Autodesk Inventor part; units mm, degrees
ref_plane "YZ Plane" through (0, 0, 0) normal (1, 0, 0) x (0, 1, 0)
ref_plane "XZ Plane" through (0, 0, 0) normal (0, 1, 0) x (-1, 0, 0)
ref_plane "XY Plane" through (0, 0, 0) normal (0, 0, 1) x (1, 0, 0)
sketch "Boceto1" plane through (0, 0, 0) normal (0, 1, 0) x (-1, 0, 0)
  circle A0 centre (0, 0) radius 15
  dimension "d0" = 30
extrude "Extrusión1" add sketch "Boceto1" along normal blind 4
sketch "Boceto2" plane through (0, 4, 0) normal (0, 1, 0) x (1, 0, 0)
  line L0 (10.3923, 6) -> (10.3923, -6)
  line L1 (10.3923, -6) -> (0, -12)
  line L2 (0, -12) -> (-10.3923, -6)
  line L3 (-10.3923, -6) -> (-10.3923, 6)
  line L4 (-10.3923, 6) -> (0, 12)
  line L5 (0, 12) -> (10.3923, 6)
  point P0 (0, 0)
  point P1 (0, 0)
  point P2 (10.3923, 0)
  dimension "d3" = 12
extrude "Extrusión2" add sketch "Boceto2" along normal blind 8
sketch "Boceto3" plane through (0, 0, 0) normal (0, -1, 0) x (1, 0, 0)
  circle A0 centre (0, 0) radius 9
  dimension "d6" = 18
extrude "Extrusión3" cut sketch "Boceto3" against normal blind 8
sketch "Boceto4" plane through (0, 12, 0) normal (0, 1, 0) x (1, 0, 0)
  circle A0 centre (0, 0) radius 3
  dimension "d9" = 6
extrude "Extrusión4" cut sketch "Boceto4" against normal up to next
properties part number "shocks_mover" material "Goma"
Could you check a few things on this model? Use its own coordinates, in mm. A direction names the side the tool comes from. Coordinates: 2 decimals unless noted, no trailing zeros. Order: outer loops, then holes, each group sorted by start corner. A loop starts at its lowest first (then second) coordinate and runs counter-clockwise, first axis right, second up. Notation, with made-up numbers: (6.5, 60.25) - (50.5, 60.25) arc R18 ccw to (50.5, 82.25) - close; hole circle Ø8 at (87.25, 33.5). An arc over 180 degrees is marked (long way). Answer in a Markdown table with one row per item. Add a question column.
(1) If we mould it in two halves opening along X, with no side actions, what happens to faces 6 (the face through (4, 4, 10)), 7 (the face through (-5.269, 7.944, -8.958)), 8 (the face through (-1.172, 3.944, 8.923)), 9 (the face through (0, 8, -4))? For each: released by +X, released by -X, zero draft, split by the parting line, or undercut.
(2) On a 3-axis mill with a long thin cutter (end or side, diameter ignored), from which of +Z, -Z, +X, -X, +Y, -Y can I reach the whole of each face in a straight line? I mean faces 1 (the face through (5.123, 7.944, -9.042)), 2 (the face through (-10.392, 8, 0)), 3 (the face through (10.392, 8, 0)), 4 (the face through (-5.123, 7.944, 9.042)), 5 (the face through (5.269, 7.944, 8.958)). Say none if no direction works.
(3) If we section it at A-A, the plane z = 0: Please give me the cut outline in (x, y).
(4) If we section it at C-C, the plane x = 1.5: Please give me the cut outline in (y, z), then the cut area to 3 significant figures.
(5) I need wall thicknesses on L1, parallel to X at y = 10.25, z = 0; L2, parallel to Z at x = 0, y = 11.25; L3, parallel to Z at x = 0, y = 3.75. Which ranges of each line are inside material? Lowest first, please.
(6) If we section it at B-B, the plane y = 6: Please give me the cut outline in (x, z).
(7) Will these pins go through, and if not, where does the flat tip stop? pin 1 (16 mm diameter, centred on x = 0, z = 0, fed in from +Y); pin 2 (5 mm diameter, centred on x = 0, z = 0, fed in from +Y); pin 3 (4 mm diameter, centred on y = 9.5, z = 0, fed in from -X); pin 4 (1.5 mm diameter, centred on x = -6, y = 5.5, fed in from -Z).
(8) If we section it at D-D, the plane y = 11: Please give me the cut outline in (x, z).
Results are:
| question | item | result |
|---|---|---|
| 1 | face 6 | zero draft |
| 1 | face 7 | released by -X |
| 1 | face 8 | undercut |
| 1 | face 9 | undercut |
| 2 | face 1 | -Z, +X, +Y |
| 2 | face 2 | +Z, -Z, -X, +Y |
| 2 | face 3 | +Z, -Z, +X, +Y |
| 2 | face 4 | +Z, -X, +Y |
| 2 | face 5 | +Z, +X, +Y |
| 3 | outline | (-15, 0) - (-9, 0) - (-9, 8) - (-3, 8) - (-3, 12) - (-10.39, 12) - (-10.39, 4) - (-15, 4) - close; (3, 8) - (9, 8) - (9, 0) - (15, 0) - (15, 4) - (10.39, 4) - (10.39, 12) - (3, 12) - close |
| 4 | outline | (0, -14.92) - (4, -14.92) - (4, -11.13) - (12, -11.13) - (12, -2.6) - (8, -2.6) - (8, -8.87) - (0, -8.87) - close; (0, 8.87) - (8, 8.87) - (8, 2.6) - (12, 2.6) - (12, 11.13) - (4, 11.13) - (4, 14.92) - (0, 14.92) - close |
| 4 | area | 135 mm2 |
| 5 | L1 | x = -10.39 to -3, 3 to 10.39 |
| 5 | L2 | z = -12 to -3, 3 to 12 |
| 5 | L3 | z = -15 to -9, 9 to 15 |
| 6 | outline | (-10.39, -6) - (0, -12) - (10.39, -6) - (10.39, 6) - (0, 12) - (-10.39, 6) - close; hole circle Ø18 at (0, 0) |
| 7 | pin 1 | stops at y = 12 |
| 7 | pin 2 | passes through |
| 7 | pin 3 | stops at x = -10.39 |
| 7 | pin 4 | stops at z = -8.97 |
| 8 | outline | (-10.39, -6) - (0, -12) - (10.39, -6) - (10.39, 6) - (0, 12) - (-10.39, 6) - close; hole circle Ø6 at (0, 0) |
